from build123d import *

# Parameters (mm, degrees)
EXTRUDE1_DEPTH = 3
SKETCH2_R      = 4
EXTRUDE2_DEPTH = 9.5
SKETCH3_R      = 3
EXTRUDE3_DEPTH = 11.5
SKETCH4_R      = 1.5
EXTRUDE4_DEPTH = 24
SKETCH5_R      = 1.5
EXTRUDE5_DEPTH = 3


with BuildPart() as part:
    # Sketch1 → Extrude1 (new body)
    with BuildSketch(Plane.XY):
        with BuildLine():
            Line((10, 4), (0, 4))
            ThreePointArc((0, 4), (-2.828427125, 2.828427125), (-4, 0))
            Line((-4, 0), (-4, -10))
            ThreePointArc((-4, -10), (5.899494937, -5.899494937), (10, 4))
        make_face()
    extrude(amount=EXTRUDE1_DEPTH)

    # Sketch2 → Extrude2 (add)
    with BuildSketch(Plane.XY.offset(3)):
        with Locations(Location((0, 0, 0), (0, 0, 180))):
            Circle(SKETCH2_R)
    extrude(amount=EXTRUDE2_DEPTH)

    # Sketch3 → Extrude3 (add)
    with BuildSketch(Plane.XY.offset(12.5)):
        Circle(SKETCH3_R)
    extrude(amount=EXTRUDE3_DEPTH)

    # Sketch4 → Extrude4 (cut)
    with BuildSketch(Plane.XY.offset(24)):
        Circle(SKETCH4_R)
    extrude(amount=-EXTRUDE4_DEPTH, mode=Mode.SUBTRACT)

    # Sketch5 → Extrude5 (cut)
    with BuildSketch(Plane.XY.offset(3)):
        with Locations((7, 1)):
            Circle(SKETCH5_R)
        with Locations((-1, -7)):
            Circle(SKETCH5_R)
    extrude(amount=-EXTRUDE5_DEPTH, mode=Mode.SUBTRACT)


solid = part.part
Could you check a few things on this model? Use its own coordinates, in mm. A direction names the side the tool comes from. Give positions to 0.01 mm unless a question says otherwise; leave off trailing zeros. Write each loop counter-clockwise with the first axis right and the second up, starting at its lowest first coordinate (ties: lowest second). Pieces come first, ordered by that corner, then holes. Notation, with made-up numbers: (33.25, -28) -> (84.25, -28) arc R19 cw to (84.25, -21) -> close; hole circle Ø5 at (40, 61.5). An arc over 180 degrees is marked (long way). Answer as CSV lines item,"result". Start each with the question number.
(1) If we section it at C-C, the plane y = -1.25: Write out the boundary of the cut face in (x, z).
(2) I'm going to push flat-ended pins straight in: pin 1 Ø4 at (x, y) = (5.5, -7) entering from +Z; pin 2 Ø2 at (y, z) = (-4.5, 11.5) entering from -X; pin 3 Ø2 at (y, z) = (-1, 15.5) entering from -X. Where does each tip first touch, or does it pass through?
(3) Which directions (+Z, -Z, +X, -X, +Y, -Y) give clear straight access to the entire face, cutting with the end or side of a thin tool? Please do faces 1 (the face through (1.3, -1.3, 24)), 2 (the face through (-1, -3, 12.5)).
(4) If we section it at A-A, the plane x = -1.25: Write out the boundary of the cut face in (y, z).
(5) If we section it at B-B, the plane y = 1: Write out the boundary of the cut face in (x, z).
(6) If we mould it in two halves opening along Y, with no side actions, what happens to faces 3 (the face through (-4, -5, 1)), 4 (the face through (-3, 0, 18)), 5 (the face through (5.8, -6, 1.5)), 6 (the face through (-1.325, -8.464, 1.521))? For each: +Y half, -Y half, draft (parallel to the pull), parting line (faces both ways), or undercut.
(7) Please list where these lines run through material, in increasing order: line 1 (Y direction, x = -1, z = 1); line 2 (Z direction, x = -0.5, y = -3.5); line 3 (X direction, y = -8.25, z = 2.5).
(8) If we section it at D-D, the plane x = 0.75: Write out the boundary of the cut face in (y, z).
Answer list:
1,outline,"(-4, 0) -> (-0.83, 0) -> (-0.83, 24) -> (-2.73, 24) -> (-2.73, 12.5) -> (-3.8, 12.5) -> (-3.8, 3) -> (-4, 3) -> close; (0.83, 0) -> (8.98, 0) -> (8.98, 3) -> (3.8, 3) -> (3.8, 12.5) -> (2.73, 12.5) -> (2.73, 24) -> (0.83, 24) -> close"
2,pin 1,"z = 3"
2,pin 2,"x = -1.94"
2,pin 3,"x = -3"
3,face 1,"+Z, +X, -X, +Y, -Y"
3,face 2,"+Z"
4,outline,"(-9.73, 0) -> (-8.48, 0) -> (-8.48, 3) -> (-9.73, 3) -> close; (-5.52, 0) -> (-0.83, 0) -> (-0.83, 24) -> (-2.73, 24) -> (-2.73, 12.5) -> (-3.8, 12.5) -> (-3.8, 3) -> (-5.52, 3) -> close; (0.83, 0) -> (3.8, 0) -> (3.8, 12.5) -> (2.73, 12.5) -> (2.73, 24) -> (0.83, 24) -> close"
5,outline,"(-3.87, 0) -> (-1.12, 0) -> (-1.12, 24) -> (-2.83, 24) -> (-2.83, 12.5) -> (-3.87, 12.5) -> close; (1.12, 0) -> (5.5, 0) -> (5.5, 3) -> (3.87, 3) -> (3.87, 12.5) -> (2.83, 12.5) -> (2.83, 24) -> (1.12, 24) -> close; (8.5, 0) -> (9.67, 0) -> (9.67, 3) -> (8.5, 3) -> close"
6,face 3,"draft"
6,face 4,"parting line"
6,face 5,"-Y half"
6,face 6,"undercut"
7,line 1,"-9.67 to -8.5, -5.5 to -1.12, 1.12 to 3.87"
7,line 2,"0 to 12.5"
7,line 3,"-4 to -1.83, -0.17 to 2.78"
8,outline,"(-9.17, 0) -> (-1.3, 0) -> (-1.3, 24) -> (-2.9, 24) -> (-2.9, 12.5) -> (-3.93, 12.5) -> (-3.93, 3) -> (-9.17, 3) -> close; (1.3, 0) -> (4, 0) -> (4, 3) -> (3.93, 3) -> (3.93, 12.5) -> (2.9, 12.5) -> (2.9, 24) -> (1.3, 24) -> close"
